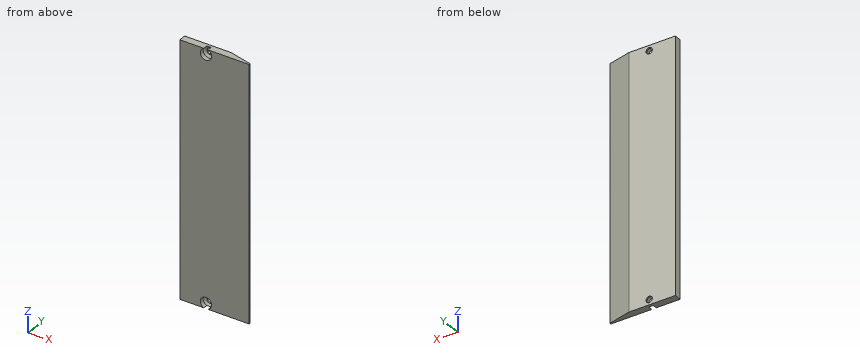
```python
from build123d import *

# Parameters (mm, degrees)
BOSS_EXTRUDE1_DEPTH = 44.5
HOLEWZD2_AT_2_COUNT = 2
HOLEWZD2_AT_2_PITCH = 85.3


with BuildPart() as part:
    # Sketch1 → Boss-Extrude1 (new, symmetric)
    with BuildSketch(Plane.XY):
        Polygon((0, 0), (0, 2.5), (16.278438133, 2.5), (24.3, 0.5), (24.3, 0), align=None)
    extrude(amount=BOSS_EXTRUDE1_DEPTH, both=True)

    # Sketch6 → HoleWzd2 (revolve, cut)
    with BuildSketch(Plane(origin=(9.15, 0, 42.65), x_dir=(0, 0, -1), z_dir=(1, 0, 0))):
        Polygon((0, 0), (0, 2.5), (1.1, 2.5), (1.1, 2.040774557), (2, 1.5), (2, 0), align=None)
    holewzd2 = revolve(axis=Axis((9.15, -6.130023899, 42.65), (0, 1, 0)), mode=Mode.SUBTRACT)

    # HoleWzd2 at 2: HoleWzd2 ×2
    with Locations(*[(0, 0, -i * HOLEWZD2_AT_2_PITCH) for i in range(1, HOLEWZD2_AT_2_COUNT)]):
        add(holewzd2, mode=Mode.SUBTRACT)


solid = part.part
```
Can you work these out from the model? Positions are in its coordinate system, mm. Give positions to 0.01 mm unless a question says otherwise; leave off trailing zeros. Loops run counter-clockwise (first coordinate to the right, second up) from the corner with the lowest first, then second, coordinate; pieces in that order, holes last. Notation, with made-up numbers: M 2,33 L 15,33 A27 ccw 15,51 Z; hole C 80.5,-23.5 d1. An arc over 180 degrees is marked long. One line per question, with ' | ' between items. Start each with the question number.
Q1. If I drill on line 1 (Z direction, x = 9.15, y = 2.15); line 2 (Z direction, x = 9.15, y = 0.9); line 3 (Y direction, x = 22.5, z = -21.5), over which ranges is the centre line in solid material (lowest first)? Write a range as from..to.
Q2. If we section it at D-D (y = 1.05): Please give me the cut outline in (x, z), plus the area to 3 significant figures.
Q3. For pin 1 Ø1 at (x, z) = (21, -32) entering from +Y, with a flat end and sliding along its axis, tell me the tip position at first contact or that it passes through.
Q4. If we section it at A-A (z = 42.65): Please give me the cut outline in (x, y).
Q5. If we section it at B-B (x = 9.15): Please give me the cut outline in (y, z), plus the area to 3 significant figures.
Q6. If we section it at C-C (z = -1.5): Please give me the cut outline in (x, y).
Computed:
1) line 1: z = -44.5..-43.75, -41.55..41.55, 43.75..44.5 | line 2: z = -40.65..40.65 | line 3: y = 0..0.95
2) outline: M 0,-44.5 L 8.39,-44.5 A2 cw long 9.91,-44.5 L 22.09,-44.5 L 22.09,44.5 L 9.91,44.5 A2 cw long 8.39,44.5 L 0,44.5 Z | area: 1,940 mm²
3) pin 1: stops at y = 1.45
4) outline: M 0,0 L 7.15,0 L 7.15,1.5 L 8.05,2.04 L 8.05,2.5 L 0,2.5 Z; M 10.25,2.04 L 11.15,1.5 L 11.15,0 L 24.3,0 L 24.3,0.5 L 16.28,2.5 L 10.25,2.5 Z
5) outline: M 0,-40.65 L 1.5,-40.65 L 2.04,-41.55 L 2.5,-41.55 L 2.5,41.55 L 2.04,41.55 L 1.5,40.65 L 0,40.65 Z; M 1.59,-44.5 L 2.5,-44.5 L 2.5,-43.75 L 2.04,-43.75 Z; M 1.59,44.5 L 2.04,43.75 L 2.5,43.75 L 2.5,44.5 Z | area: 206 mm²
6) outline: M 0,0 L 24.3,0 L 24.3,0.5 L 16.28,2.5 L 0,2.5 Z
